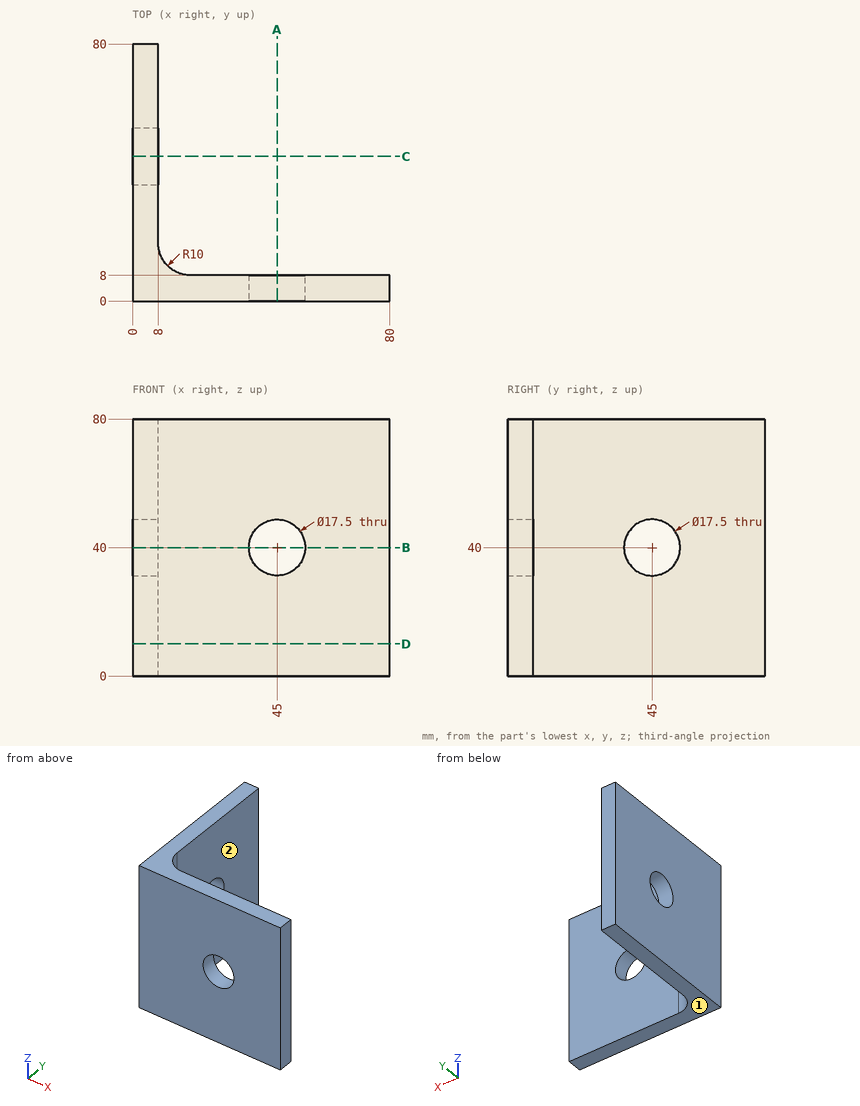
Here's the drawing with two shaded views (mm, measured from the low corner). I have some questions. A direction names the side the tool comes from. Coordinates: 2 decimals unless noted, no trailing zeros. Order: outer loops, then holes, each group sorted by start corner. A loop starts at its lowest first (then second) coordinate and runs counter-clockwise, first axis right, second up.
Item 1: If we section it at B-B on z = 40: List the corners of the cut face in (x, y) for me.
Result sheet:
outline: (0, 0) - (36.25, 0) - (36.25, 8) - (18, 8) arc R10 cw to (8, 18) - (8, 36.25) - (0, 36.25) - close; (0, 53.75) - (8, 53.75) - (8, 80) - (0, 80) - close; (53.75, 0) - (80, 0) - (80, 8) - (53.75, 8) - close
Item 2: For the marked faces 1 and 2, which set-ups out of +Z, -Z, +X, -X, +Y, -Y let a thin tool reach every point of the face, with its end or its side?
Result sheet:
face 1: -Z, +X, -X, +Y, -Y
face 2: +Z, -Z, +X, +Y
Item 3: I need wall thicknesses on line 1 (Z direction, x = 2.5, y = 45); line 2 (X direction, y = 68, z = 51.5). Which ranges of each line are inside material? Lowest first, please.
Result sheet:
line 1: z = 0 to 31.25, 48.75 to 80
line 2: x = 0 to 8
Item 4: For P1, Ø12, axis at y = 71, z = 9, coming from the +X side; P2, Ø2, axis at x = 37.5, z = 27.5, coming from the +Y side, each with a flat end and sliding along its axis, tell me the tip position at first contact or that it passes through.
Result sheet:
P1: stops at x = 8
P2: stops at y = 8
Item 5: If we section it at D-D on z = 10: List the corners of the cut face in (x, y) for me, plus the area to 3 significant figures.
Result sheet:
outline: (0, 0) - (80, 0) - (80, 8) - (18, 8) arc R10 cw to (8, 18) - (8, 80) - (0, 80) - close
area: 1,240 mm2
Item 6: If we section it at A-A on x = 45: List the corners of the cut face in (y, z) for me.
Result sheet:
outline: (0, 0) - (8, 0) - (8, 31.25) - (0, 31.25) - close; (0, 48.75) - (8, 48.75) - (8, 80) - (0, 80) - close
